Part model, mm, in its own coordinate system. Give positions to 0.01 mm unless a question says otherwise; leave off trailing zeros. Order: outer loops, then holes, each group sorted by start corner. A loop starts at its lowest first (then second) coordinate and runs counter-clockwise, first axis right, second up.
1. Probe line 1 (X direction, y = 1.85, z = -42.5); line 2 (Z direction, x = 23.5, y = 2.5); line 3 (Z direction, x = 25, y = 2.4). List the from-to ranges inside material, lowest first.
2. Slice it at B-B on z = -35.5. List the corners of the cut face in (x, y), and give its area (3 significant figures).
3. Slice it at A-A on y = 3.1. List the corners of the cut face in (x, z).
4. Drop flat-ended pins along their axis: pin 1 Ø1.5 at (x, y) = (39, 2.5) entering from -Z; pin 2 Ø8 at (x, z) = (28.5, -15) entering from -Y. Give the stop position or say it passes through.
5. Slice it at C-C on x = 37.5. List the corners of the cut face in (y, z), and give its area (3 significant figures).
from build123d import *

# Parameters (mm, degrees)
EXTRUDE_1_DEPTH = 4
FILLET_1_R      = 8


with BuildPart() as part:
    # 草图1 → 凸台-拉伸1 (new body)
    with BuildSketch(Plane(origin=(0, 0, 0), x_dir=(1, 0, 0), z_dir=(0, 1, 0))):
        Polygon((0, 0), (60, 0), (0, 60), align=None)
    extrude(amount=EXTRUDE_1_DEPTH)

    # 圆角1
    fillet_1_edges = [part.edges().sort_by_distance(p)[0] for p in [
        (0, 2, -60),
        (60, 2, 0),
        (0, 2, 0),
    ]]
    fillet(fillet_1_edges, radius=FILLET_1_R)


solid = part.part
Data:
1. line 1: x = 0.21 to 17.5
1. line 2: z = -36.5 to 0
1. line 3: z = -35 to 0
2. outline: (0, 0) - (24.5, 0) - (24.5, 4) - (0, 4) - close
2. area: 98.0 mm2
3. outline: (0, -40.69) arc R8 ccw to (13.66, -46.34) - (46.34, -13.66) arc R8 ccw to (40.69, 0) - (8, 0) arc R8 ccw to (0, -8) - close
4. pin 1: stops at z = -21.75
4. pin 2: stops at y = 0
5. outline: (0, -22.5) - (4, -22.5) - (4, 0) - (0, 0) - close
5. area: 90.0 mm2
